```python
from build123d import *

# Parameters (mm, degrees)
EXTRUDE_1_DEPTH     = 60
EXTRUDE_2_DEPTH     = 5
SKETCH_4_R          = 1.6
CUT_EXTRUDE_1_DEPTH = 158.885383869
EXTRUDE_3_DEPTH     = 4
EXTRUDE_4_DEPTH     = 4
SKETCH_7_R          = 5
CUT_EXTRUDE_2_DEPTH = 158.885383869


with BuildPart() as part:
    # 草图1 → 凸台-拉伸1 (new body)
    with BuildSketch(Plane.XY):
        with BuildLine():
            Line((-100, 0), (-103, 0))
            ThreePointArc((-103, 0), (-96.158783929, -36.911898803), (-76.543917024, -68.920452455))
            Line((-76.543917024, -68.920452455), (-74.314482548, -66.913060636))
            ThreePointArc((-74.314482548, -66.913060636), (-93.35804265, -35.836794955), (-100, 0))
        make_face()
    extrude(amount=EXTRUDE_1_DEPTH)

    # 草图2 → 凸台-拉伸2 (add)
    with BuildSketch(Plane.XY.offset(60)):
        with BuildLine():
            Line((-75.335122837, -67.83204928), (-91.406813534, -82.303064582))
            ThreePointArc((-91.406813534, -82.303064582), (-114.830392459, -44.079257794), (-123, 0))
            Line((-123, 0), (-101.373406978, 0))
            ThreePointArc((-101.373406978, 0), (-94.640228522, -36.328979997), (-75.335122837, -67.83204928))
        make_face()
    extrude(amount=-EXTRUDE_2_DEPTH)

    # 草图4 → 切除-拉伸1 (cut, through all)
    with BuildSketch(Plane(origin=(0, 0, 55), x_dir=(-1, 0, 0), z_dir=(0, 0, -1))):
        with Locations((97.525531058, -60.940715387)):
            Circle(SKETCH_4_R)
        with Locations((106.626143275, -43.079758243)):
            Circle(SKETCH_4_R)
    extrude(amount=-CUT_EXTRUDE_1_DEPTH, mode=Mode.SUBTRACT)

    # 草图5 → 凸台-拉伸3 (add)
    with BuildSketch(Plane(origin=(0, 0, 0), x_dir=(1, 0, 0), z_dir=(0, 1, 0))):
        Polygon((-103, 0), (-123, -55), (-100, -55), (-100, 0), align=None)
    extrude(amount=-EXTRUDE_3_DEPTH)

    # 草图6 → 凸台-拉伸4 (add)
    with BuildSketch(Plane(origin=(0, 0, 0), x_dir=(0, 0, -1), z_dir=(0.6691306063588633, -0.7431448254773898, 0))):
        Polygon((-55, -123), (0, -103), (0, -100), (-55, -100), align=None)
    extrude(amount=-EXTRUDE_4_DEPTH)

    # 草图7 → 切除-拉伸2 (cut, through all)
    with BuildSketch(Plane(origin=(0, 0, 55), x_dir=(-1, 0, 0), z_dir=(0, 0, -1))):
        with Locations((107.624346688, -9)):
            Circle(SKETCH_7_R)
    extrude(amount=-CUT_EXTRUDE_2_DEPTH, mode=Mode.SUBTRACT)


solid = part.part
```
Source: CAD feature listing. Evaluate the final solid. Frame: model axes, mm. A direction names the side the tool comes from. Round coordinates to 2 decimals unless told otherwise and drop trailing zeros. Order: outer loops, then holes, each group sorted by start corner. A loop starts at its lowest first (then second) coordinate and runs counter-clockwise, first axis right, second up. Notation, with made-up numbers: (50.5, 77.25) -> (105.5, 77.25) arc R33 ccw to (105.5, 111.25) -> close; hole circle Ø10 at (24, -34). An arc over 180 degrees is marked (long way). One line per item, written item: value. Start each with the question number.
Q1. Draft query along X for faces 4 (the cylindrical face through (-112.393, -7.498, 57.465)), 5 (the flat face through (-85.399, -74.24, 27.885)), 6 (the flat face through (-94, -35, 0)). Return one class per face: pulls with the +X half, pulls with the -X half, needs draft (parallel to the pull), parting line crosses it, or undercut.
Q2. Section query A-A (y = -11). Return the cut outline in (x, z).
Q3. Access query for faces 1 (the flat face through (-112.86, -1.97, 27.12)), 2 (the cylindrical face through (-96.327, -36.47, 27.115)), 3 (the flat face through (-109, -4, 39)). Directions: +Z, -Z, +X, -X, +Y, -Y. A direction counts if a zero-diameter tool reaches every point of the face in a straight line with its end or side. Return the directions, or none.
Q4. Section query D-D (x = -95). Return the cut outline in (y, z), plus the area to 3 significant figures.
Q5. Material intervals for probe 1 along Y at (x, z) = (-109, 44); probe 2 along Z at (x, y) = (-120, -19); probe 3 along Y at (x, z) = (-91, 48), sorted ascending.
Q6. Pin query (flat end, axial travel): pin 1 (2 mm diameter, centred on y = -27.5, z = 41.5, fed in from -X); pin 2 (6 mm diameter, centred on y = -19, z = 46, fed in from +X); pin 3 (1 mm diameter, centred on y = -52.5, z = 38.5, fed in from -X); pin 4 (5 mm diameter, centred on x = -97.53, y = -60.94, fed in from +Z). Return the tip coordinate at first contact, or that it passes through.
Q7. Section query B-B (z = 22.5). Return the cut outline in (x, y), plus the area to 3 significant figures.
Q8. Section query C-C (x = -84). Return the cut outline in (y, z).
Findings below:
1. face 4: undercut
1. face 5: pulls with the -X half
1. face 6: needs draft
2. outline: (-122.51, 55) -> (-112.21, 55) -> (-112.21, 60) -> (-122.51, 60) -> close; (-103.04, 55) -> (-102.41, 55) -> (-102.41, 0) -> (-99.39, 0) -> (-99.39, 60) -> (-103.04, 60) -> close
3. face 1: -Z, -X, +Y, -Y
3. face 2: -Z, -X
3. face 3: -Z, -X, -Y
4. outline: (-78.13, 55) -> (-39.8, 55) -> (-39.8, 0) -> (-31.22, 0) -> (-31.22, 60) -> (-78.13, 60) -> close
4. area: 706 mm²
5. probe 1: -4 to 0
5. probe 2: 55 to 60
5. probe 3: -78.95 to -76.55, -48.25 to -41.46
6. pin 1: x = -99.53
6. pin 2: x = -97.55
6. pin 3: x = -88.91
6. pin 4: z = 60
7. outline: (-111.18, -4) -> (-102.92, -4) arc R103 ccw to (-79.16, -65.9) -> (-85.3, -71.42) -> (-82.62, -74.4) -> (-74.31, -66.91) arc R100 cw to (-100, 0) -> (-111.18, 0) -> close
7. area: 289 mm²
8. outline: (-75.63, 27.59) -> (-70.25, 17.69) -> (-70.25, 55) -> (-59.61, 55) -> (-59.61, 0) -> (-54.26, 0) -> (-54.26, 60) -> (-75.63, 60) -> close
